Input: dimensioned drawing with shaded views. Units: mm. Origin: part minimum x, y, z. A direction names the side the tool comes from. Give positions to 0.01 mm unless a question says otherwise; leave off trailing zeros. Write each loop counter-clockwise with the first axis right and the second up, starting at its lowest first coordinate (ties: lowest second). Pieces come first, ordered by that corner, then holes. Notation, with made-up numbers: (58.25, -34.5) - (76.25, -34.5) arc R31 ccw to (76.25, 4.5) - close; hole circle Ø2 at (30.25, -36). An arc over 180 degrees is marked (long way). Answer as CSV lines item,"result".
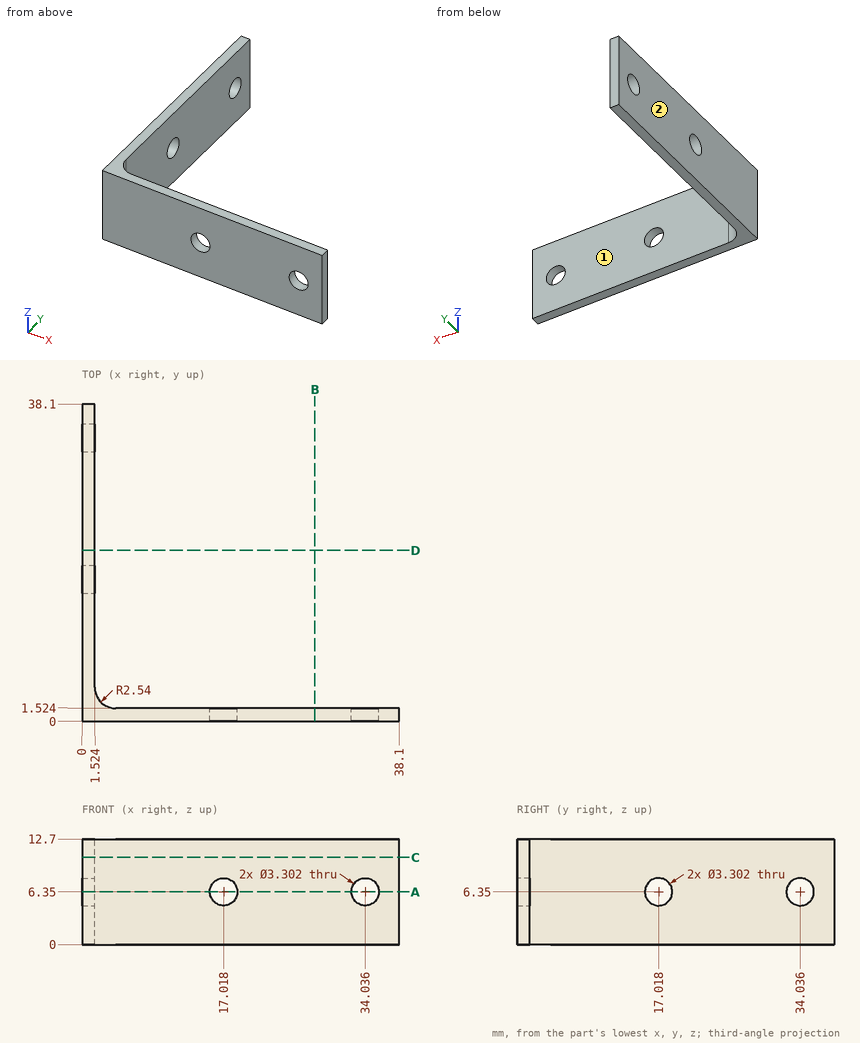
Item 1: Cut plane B-B on x = 28. Return the cut outline in (y, z).
The answers:
outline,"(0, 0) - (1.52, 0) - (1.52, 12.7) - (0, 12.7) - close"
Item 2: Contact query for flat-ended pins moving along their axis: pin 1 (4.5 mm diameter, centred on y = 34.036, z = 6.35, fed in from +X); pin 2 (2 mm diameter, centred on x = 29, z = 10, fed in from +Y); pin 3 (4 mm diameter, centred on x = 34.036, z = 6.35, fed in from -Y). Output: stop coordinate, or through.
The answers:
pin 1,"x = 1.52"
pin 2,"y = 1.52"
pin 3,"y = 0"
Item 3: Reachability of the marked faces 1 and 2 from +Z, -Z, +X, -X, +Y, -Y: full face, straight path, thin tool, end or side. Return the list, or none.
The answers:
face 1,"+Z, -Z, +X, +Y"
face 2,"+Z, -Z, -X, +Y, -Y"
Item 4: Cut plane C-C on z = 10.5. Return the cut outline in (x, y), plus the area to 3 significant figures.
The answers:
outline,"(0, 0) - (38.1, 0) - (38.1, 1.52) - (4.06, 1.52) arc R2.54 cw to (1.52, 4.06) - (1.52, 38.1) - (0, 38.1) - close"
area,"115 mm²"
Item 5: Ray query, line 1 (X direction, y = 1, z = 6.35) (3 decimals); line 2 (X direction, y = 23.5, z = 10.75). Return the intervals inside material, ascending. Write a range as from..to.
The answers:
line 1,"0..15.367, 18.669..32.385, 35.687..38.1"
line 2,"0..1.52"
Item 6: Cut plane A-A on z = 6.35. Return the cut outline in (x, y) (3 decimals), plus the area to 3 significant figures.
The answers:
outline,"(0, 0) - (15.367, 0) - (15.367, 1.524) - (4.064, 1.524) arc R2.54 cw to (1.524, 4.064) - (1.524, 15.367) - (0, 15.367) - close; (0, 18.669) - (1.524, 18.669) - (1.524, 32.385) - (0, 32.385) - close; (0, 35.687) - (1.524, 35.687) - (1.524, 38.1) - (0, 38.1) - close; (18.669, 0) - (32.385, 0) - (32.385, 1.524) - (18.669, 1.524) - close; (35.687, 0) - (38.1, 0) - (38.1, 1.524) - (35.687, 1.524) - close"
area,"95.1 mm²"
